Check sheet for the modelled part. Datum: model origin and axes. Units: mm. A direction names the side the tool comes from. Give positions to 0.01 mm unless a question says otherwise; leave off trailing zeros. Order: outer loops, then holes, each group sorted by start corner. A loop starts at its lowest first (then second) coordinate and runs counter-clockwise, first axis right, second up.
```python
from build123d import *

# Parameters (mm, degrees)
F0_W      = 100
F0_H      = 70
F1_DEPTH  = 30
F2_W      = 5
F2_H      = 70
F3_DEPTH  = 30
F4_W      = 12
F4_H      = 22.185914
F4_H_2    = 22.385787
F5_DEPTH  = 5
F6_W      = 5
F6_H      = 70
F7_DEPTH  = 20
F8_R      = 2
F9_W      = 74.35465
F9_H      = 61.962207
F10_DEPTH = 2


with BuildPart() as f1:
    # F0 (on Top) → F1 (new body)
    with BuildSketch(Plane.XY):
        with Locations((50, 35)):
            Rectangle(F0_W, F0_H)
    extrude(amount=F1_DEPTH)

    # F2 (on face) → F3 (join)
    with BuildSketch(Plane.XY.offset(30)):
        with Locations((97.5, 35)):
            Rectangle(F2_W, F2_H)
    extrude(amount=F3_DEPTH)

    # F4 (on face) → F5 (join)
    with BuildSketch(Plane.XY.offset(30)):
        with Locations((89, 23.784902)):
            Rectangle(F4_W, F4_H)
        with Locations((89, 53.665931)):
            Rectangle(F4_W, F4_H_2)
    extrude(amount=F5_DEPTH)

    # F6 (on face) → F7 (join)
    with BuildSketch(Plane.XY.offset(30)):
        with Locations((2.5, 35)):
            Rectangle(F6_W, F6_H)
    extrude(amount=F7_DEPTH)

    # F8
    f8_edges = [f1.edges().sort_by_distance(p)[0] for p in [
        (83, 23.784902, 35),
        (89, 12.691945, 35),
        (89, 34.877859, 35),
        (83, 53.66593, 35),
        (89, 42.473037, 35),
        (89, 64.858824, 35),
        (50, 0, 30),
        (50, 70, 30),
        (2.5, 0, 50),
        (2.5, 70, 50),
        (97.5, 0, 60),
        (97.5, 70, 60),
        (95, 35, 60),
        (100, 35, 60),
        (5, 35, 50),
        (0, 35, 50),
    ]]
    fillet(f8_edges, radius=F8_R)

    # F9 (on face) → F10 (join)
    with BuildSketch(Plane.XY.offset(30)):
        with Locations((43.801598, 35.36119)):
            Rectangle(F9_W, F9_H)
    extrude(amount=F10_DEPTH)


solid = f1.part
```
(1) Gauge pin test, flat ends, axial feed: pin 1 Ø0.9 at (x, z) = (91, 31) entering from +Y; pin 2 Ø3 at (x, y) = (70, 10.5) entering from +Z; pin 3 Ø2 at (y, z) = (12, 49.5) entering from -X. Record the tip position at first contact, or that the pin passes through.
Response values:
pin 1: stops at y = 64.86
pin 2: stops at z = 32
pin 3: stops at x = 0.06
(2) Cross-section at B-B on y = 28.5. Enter the section's corners in (x, z).
Response values:
outline: (0, 0) - (100, 0) - (100, 58) arc R2 ccw to (98, 60) - (97, 60) arc R2 ccw to (95, 58) - (95, 35) - (85, 35) arc R2 ccw to (83, 33) - (83, 30) - (80.98, 30) - (80.98, 32) - (6.62, 32) - (6.62, 30) - (5, 30) - (5, 48) arc R2 ccw to (3, 50) - (2, 50) arc R2 ccw to (0, 48) - close
(3) Cross-section at A-A on z = 44. Enter the section's corners in (x, y), then the cut area to 3 significant figures.
Response values:
outline: (0, 0) - (5, 0) - (5, 70) - (0, 70) - close; (95, 0) - (100, 0) - (100, 70) - (95, 70) - close
area: 700 mm2
(4) Material ranges on L1, parallel to X at y = 40, z = 48; L2, parallel to Z at x = 26.5, y = 20; L3, parallel to Z at x = 89, y = 26.5, recorded low to high.
Response values:
L1: x = 0 to 5, 95 to 100
L2: z = 0 to 32
L3: z = 0 to 35
(5) Cross-section at C-C on x = 66.5. Enter the section's corners in (y, z).
Response values:
outline: (0, 0) - (70, 0) - (70, 28) arc R2 ccw to (68, 30) - (66.34, 30) - (66.34, 32) - (4.38, 32) - (4.38, 30) - (2, 30) arc R2 ccw to (0, 28) - close
(6) Set-up check for faces 1 (the face through (89, 12.692, 31)), 2 (the face through (89, 34.878, 31)), 3 (the face through (89, 64.859, 31)), 4 (the face through (90, 54, 35)): record each of +Z, -Z, +X, -X, +Y, -Y from which the full face is reachable in a straight line by a thin tool's end or side.
Response values:
face 1: +Z, -Y
face 2: +Z
face 3: +Z, +Y
face 4: +Z, +Y, -Y
